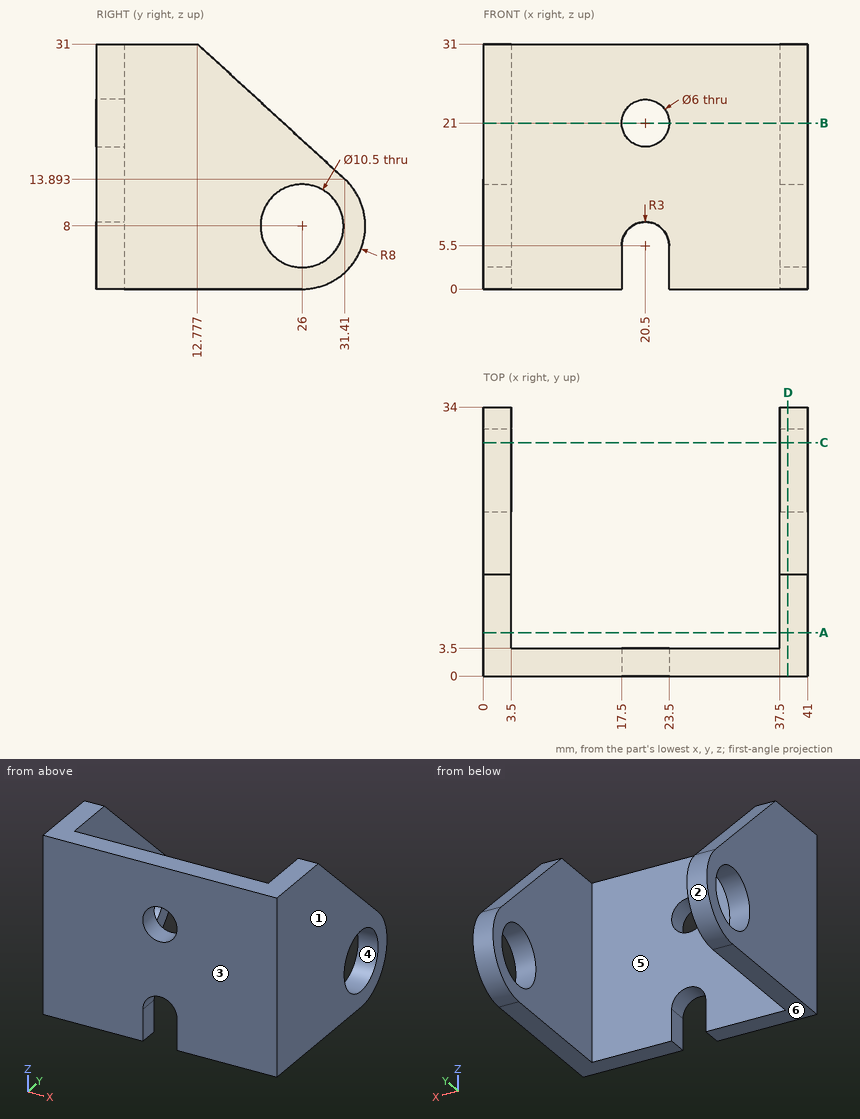
The figure shows three views and two pictorial views of one solid part (mm, origin at its lowest corner). Answer the questions. A direction names the side the tool comes from. Give positions to 0.01 mm unless a question says otherwise; leave off trailing zeros. Write each loop counter-clockwise with the first axis right and the second up, starting at its lowest first coordinate (ties: lowest second). Pieces come first, ordered by that corner, then holes. Notation, with made-up numbers: (41, -39) -> (94, -39) arc R19 cw to (94, -35) -> close; hole circle Ø11 at (31.25, -11). An arc over 180 degrees is marked (long way). Answer as a JSON object with one key per item and string values.
1) A tool of negligible diameter and unlimited length cuts with its end or side. For the marked faces 5 and 6, from which of +Z, -Z, +X, -X, +Y, -Y can it reach the whole face along a straight path? Write none if from no direction.
Findings below:
{"face 5": "+Z, -Z, +Y", "face 6": "-Z, +X, -X, +Y, -Y"}
2) Section B-B on z = 21 is taken. Write down the section's boundary in (x, y).
Findings below:
{"outline": "(0, 0) -> (17.5, 0) -> (17.5, 3.5) -> (3.5, 3.5) -> (3.5, 23.67) -> (0, 23.67) -> close; (23.5, 0) -> (41, 0) -> (41, 23.67) -> (37.5, 23.67) -> (37.5, 3.5) -> (23.5, 3.5) -> close"}
3) Section C-C on y = 29.5 is taken. Write down the section's boundary in (x, z), then the cut area to 3 significant figures.
Findings below:
{"outline": "(0, 0.81) -> (3.5, 0.81) -> (3.5, 4.09) -> (0, 4.09) -> close; (0, 11.91) -> (3.5, 11.91) -> (3.5, 15.65) -> (0, 15.65) -> close; (37.5, 0.81) -> (41, 0.81) -> (41, 4.09) -> (37.5, 4.09) -> close; (37.5, 11.91) -> (41, 11.91) -> (41, 15.65) -> (37.5, 15.65) -> close", "area": "49.1 mm^2"}
4) Flat-ended cylindrical pins translate along their axes: pin 1 Ø12 at (x, z) = (8, 17) entering from -Y; pin 2 Ø10 at (x, z) = (17.5, 16) entering from +Y. Find the tip coordinate at first contact, or state that the pin passes through.
Findings below:
{"pin 1": "stops at y = 0", "pin 2": "stops at y = 3.5"}
5) For a pull along Y with two mould halves and no side action, classify the marked faces 1, 2, 3 and 4 as pulls with the +Y half, pulls with the -Y half, needs draft (parallel to the pull), parting line crosses it, or undercut.
Findings below:
{"face 1": "needs draft", "face 2": "pulls with the +Y half", "face 3": "pulls with the -Y half", "face 4": "undercut"}
6) Section A-A on y = 5.5 is taken. Write down the section's boundary in (x, z).
Findings below:
{"outline": "(0, 0) -> (3.5, 0) -> (3.5, 31) -> (0, 31) -> close; (37.5, 0) -> (41, 0) -> (41, 31) -> (37.5, 31) -> close"}
7) Section D-D on x = 38.5 is taken. Write down the section's boundary in (y, z).
Findings below:
{"outline": "(0, 0) -> (26, 0) arc R8 ccw to (31.41, 13.89) -> (12.78, 31) -> (0, 31) -> close; hole circle Ø10.5 at (26, 8)"}
8) Straight lines are drawn through the part: probe 1 along X at (y, z) = (18.5, 12.5); probe 2 along X at (y, z) = (1.6, 21); probe 3 along Y at (x, z) = (0.8, 8). For each, find the intervals that lie inside material, in ascending order. Write a range as from..to.
Findings below:
{"probe 1": "x = 0..3.5, 37.5..41", "probe 2": "x = 0..17.5, 23.5..41", "probe 3": "y = 0..20.75, 31.25..34"}
